from build123d import *

# Parameters (mm, degrees)
F0_W     = 190
F0_H     = 42
F1_DEPTH = 2
F3_D     = 4
F4_W     = 35
F4_H     = 10
F4_W_2   = 187
F4_H_2   = 22
F5_DEPTH = 15


with BuildPart() as f1:
    # F0 (on Front) → F1 (new body)
    with BuildSketch(Plane.XZ):
        Rectangle(F0_W, F0_H)
    extrude(amount=F1_DEPTH)

    # F3 (through all)
    with Locations(Plane.XZ.offset(2)):
        with Locations((-91.5, 14.6134020761), (-91.5, -5.3865979239), (48.5, 14.6134020761), (48.5, -5.3865979239)):
            Hole(F3_D / 2)

    # F4 (on face) → F5 (join)
    with BuildSketch(Plane.XZ.offset(2)):
        with Locations((-59.5, 14)):
            Rectangle(F4_W, F4_H)
        with Locations((0, -24)):
            Rectangle(F4_W_2, F4_H_2)
    extrude(amount=F5_DEPTH)


solid = f1.part
Geometry: final body of the model. Coordinates: model frame, mm. A direction names the side the tool comes from. Coordinates: 2 decimals unless noted, no trailing zeros. Order: outer loops, then holes, each group sorted by start corner. A loop starts at its lowest first (then second) coordinate and runs counter-clockwise, first axis right, second up. Notation, with made-up numbers: M 77,4 L 84,4 A10 cw 84,17 Z; hole C -31.5,47.25 d7. An arc over 180 degrees is marked long. One line per question, with ' | ' between items. Start each with the question number.
Item 1: Draft query along X for faces 6 (the cylindrical face through (48.93, -0.99, 12.66)), 7 (the flat face through (-42, -9, 14)), 8 (the flat face through (-77, -9, 14)). Return one class per face: released by +X, released by -X, zero draft, split by the parting line, or undercut.
Item 2: Cut plane B-B, the plane y = -13.25. Return the cut outline in (x, z), then the cut area to 3 significant figures.
Item 3: Cut plane C-C, the plane x = 30. Return the cut outline in (y, z).
Item 4: Cut plane A-A, the plane x = -91.5. Return the cut outline in (y, z), then the cut area to 3 significant figures.
Item 5: Ray query, probe 1 along Z at (x, y) = (-91.5, -0.6); probe 2 along Z at (x, y) = (-53, -2.5); probe 3 along Y at (x, z) = (-32, -25). Return the intervals inside material, ascending. Write a range as [from, to].
Item 6: Pin query (flat end, axial travel): pin 1 Ø7 at (x, z) = (-46, -31) entering from +Y; pin 2 Ø5 at (y, z) = (-8, 16.5) entering from -X; pin 3 Ø7.5 at (x, y) = (-56, -13) entering from +Z. Return the tip coordinate at first contact, or that it passes through.
Item 7: Cut plane D-D, the plane z = -26. Return the cut outline in (x, y), then the cut area to 4 significant figures.
Item 8: Set-up query: faces 1 (the flat face through (-1, -2, -28)), 2 (the flat face through (-93.5, -9, -24)), 3 (the flat face through (-60, -9, 19)), 4 (the flat face through (93.5, -9, -24)), 5 (the flat face through (-1, -9, -13)). Return all of +Z, -Z, +X, -X, +Y, -Y with unobstructed straight access to the full face (end or side cutting, diameter ignored); none if empty.
A:
1) face 6: undercut | face 7: released by +X | face 8: released by -X
2) outline: M -93.5,-35 L 93.5,-35 L 93.5,-13 L -93.5,-13 Z; M -77,9 L -42,9 L -42,19 L -77,19 Z | area: 4,460 mm2
3) outline: M -17,-35 L -2,-35 L -2,-21 L 0,-21 L 0,21 L -2,21 L -2,-13 L -17,-13 Z
4) outline: M -17,-35 L -2,-35 L -2,-21 L 0,-21 L 0,-7.39 L -2,-7.39 L -2,-13 L -17,-13 Z; M -2,-3.39 L 0,-3.39 L 0,12.61 L -2,12.61 Z; M -2,16.61 L 0,16.61 L 0,21 L -2,21 Z | area: 398 mm2
5) probe 1: z = [-21, -7.39], [-3.39, 12.61], [16.61, 21] | probe 2: z = [-35, -13], [9, 19] | probe 3: y = [-17, -2]
6) pin 1: stops at y = -2 | pin 2: stops at x = -77 | pin 3: stops at z = 19
7) outline: M -93.5,-17 L 93.5,-17 L 93.5,-2 L -93.5,-2 Z | area: 2,805 mm2
8) face 1: -Z, +X, -X, +Y | face 2: +Z, -Z, -X, -Y | face 3: +Z, +X, -X, -Y | face 4: +Z, -Z, +X, -Y | face 5: +X, -X, -Y
